Input: part model. Units: mm. Frame: model coordinates. A direction names the side the tool comes from. Round coordinates to 2 decimals unless told otherwise and drop trailing zeros. Loops run counter-clockwise (first coordinate to the right, second up) from the corner with the lowest first, then second, coordinate; pieces in that order, holes last. Notation, with made-up numbers: (-31.75, 56.25) -> (-1.75, 56.25) arc R31 cw to (-1.75, 89.25) -> close; hole circle Ø8 at (9.25, 55). An arc over 180 degrees is marked (long way). One line per question, with ' | ' between items. Start each with the question number.
Q1. Cut plane C-C on x = -23. Return loops of the section in (y, z), and give its area (3 significant figures).
Q2. Access query for faces 5 (the face through (114, 12.7, 1)), 6 (the face through (-1, 20, 38.1)), 7 (the face through (2, 0, 1)), 8 (the face through (-114, 12.7, 1)). Directions: +Z, -Z, +X, -X, +Y, -Y. A direction counts if a zero-diameter tool reaches every point of the face in a straight line with its end or side. Return the directions, or none.
Q3. Material intervals for L1, parallel to X at y = 18, z = 0 (3 decimals); L2, parallel to Z at x = 95.25, y = 15.5 (3 decimals); L3, parallel to X at y = 19, z = -41, sorted ascending.
Q4. Cut plane B-B on z = 0. Return loops of the section in (x, y) (3 decimals), and give its area (3 significant figures).
Q5. Contact query for flat-ended pins moving along their axis: P1, Ø6.5, axis at y = 17, z = -33, coming from the +X side; P2, Ø7, axis at x = 96.5, z = -1, coming from the +Y side; P3, Ø1.9, axis at x = -94.5, z = 1, coming from the +Y side; P4, Ø8.5, axis at x = -76.2, z = 38.1, coming from the +Y side. Output: stop coordinate, or through.
Q6. Mould query, pull axis X, two halves, no side actions, for faces 1 (the face through (-2, 13, 101.6)), 2 (the face through (101.6, 19, -1)), 3 (the face through (-79.45, 19.77, -41.58)), 4 (the face through (-101.6, 19, -1)). Classes: pulls with the +X half, pulls with the -X half, needs draft (parallel to the pull), parting line crosses it, or undercut.
Q7. Cut plane A-A on x = 95.25. Return loops of the section in (y, z) (3 decimals).
Autodesk Inventor part; units mm, degrees
ref_plane "YZ Plane" through (0, 0, 0) normal (1, 0, 0) x (0, 1, 0)
ref_plane "XZ Plane" through (0, 0, 0) normal (0, 1, 0) x (-1, 0, 0)
ref_plane "XY Plane" through (0, 0, 0) normal (0, 0, 1) x (1, 0, 0)
sketch "Sketch1" plane through (0, 0, 0) normal (0, 1, 0) x (-1, 0, 0)
  line L0 (127, 101.6) -> (101.6, 101.6)
  line L1 (-127, 101.6) -> (-127, -101.6)
  line L2 (-127, -101.6) -> (-101.6, -101.6)
  line L3 (127, -101.6) -> (127, 101.6)
  line L4 (127, 101.6) -> (-127, -101.6) construction
  line L5 (-127, 101.6) -> (127, -101.6) construction
  line L6 (127, -101.6) -> (101.6, -101.6)
  line L7 (101.6, -101.6) -> (101.6, 101.6)
  line L8 (101.6, 101.6) -> (127, 101.6)
  line L9 (127, 101.6) -> (127, -101.6)
  line L10 (-127, -101.6) -> (-101.6, -101.6)
  line L11 (-101.6, -101.6) -> (-101.6, 101.6)
  line L12 (-101.6, 101.6) -> (-127, 101.6)
  line L13 (-127, 101.6) -> (-127, -101.6)
  line L14 (101.6, -101.6) -> (127, -101.6)
  line L15 (101.6, 101.6) -> (-101.6, 101.6)
  line L16 (-101.6, 101.6) -> (-127, 101.6)
  line L17 (-101.6, -101.6) -> (101.6, -101.6)
  point P0 (0, 0)
  dimension "d0" = 254
  dimension "d1" = 203.2
  dimension "d2" = 25.4
  dimension "d3" = 25.4
extrude "Extrusion1" add sketch "Sketch1" along normal blind 25.4 contours L7 L17 L11 L15
extrude "Extrusion2" add sketch "Sketch1" along normal blind 12.7 contours L3 L6 L7 L0 | L11 L2 L1 L12
sketch "Sketch2" plane through (0, 25.4, 0) normal (0, 1, 0) x (1, 0, 0)
  line L0 (-76.2, -38.1) -> (76.2, -38.1)
  line L1 (76.2, -38.1) -> (76.2, 38.1)
  line L2 (76.2, 38.1) -> (-76.2, 38.1)
  line L3 (-76.2, 38.1) -> (-76.2, -38.1)
  line L4 (-76.2, -38.1) -> (76.2, 38.1) construction
  line L5 (76.2, -38.1) -> (-76.2, 38.1) construction
  circle A0 centre (-76.2, 38.1) radius 4.7625
  circle A1 centre (76.2, 38.1) radius 4.7625
  circle A2 centre (76.2, -38.1) radius 4.7625
  circle A3 centre (-76.2, -38.1) radius 4.7625
  point P0 (0, 0)
  dimension "d8" = 152.4
  dimension "d9" = 76.2
  dimension "d10" = 9.525
  dimension "d11" = 9.525
  dimension "d12" = 9.525
  dimension "d13" = 9.525
extrude "Extrusion3" cut sketch "Sketch2" against normal blind 11.43
sketch "Sketch3" plane through (0, 25.4, 0) normal (0, 1, 0) x (1, 0, 0)
  circle A0 centre (-95.25, 0) radius 3.175
  line L0 (-76.2, -33.3375) -> (-76.2, 33.3375)
  point P0 (0, 0)
  dimension "d16" = 6.35
  dimension "d17" = 19.05
extrude "Extrusion4" cut sketch "Sketch3" against normal blind 12.7
mirror "Mirror1" about plane through (0, 0, 0) normal (1, 0, 0) of "Extrusion4"
equation "\"d11\" = d10"
equation "\"d12\" = d10"
equation "\"d13\" = d10"
properties part number "Case Jig"
Results:
1) outline: (0, -101.6) -> (25.4, -101.6) -> (25.4, -38.1) -> (13.97, -38.1) -> (13.97, 38.1) -> (25.4, 38.1) -> (25.4, 101.6) -> (0, 101.6) -> close | area: 4,290 mm^2
2) face 5: +Z, -Z, +X, +Y | face 6: +Y | face 7: +Z, -Z, +X, -X, -Y | face 8: +Z, -Z, -X, +Y
3) L1: -101.6 to -98.425, -92.075 to -76.2, 76.2 to 92.075, 98.425 to 101.6 | L2: -101.6 to -3.175, 3.175 to 101.6 | L3: -101.6 to -79.98, -72.42 to 72.42, 79.98 to 101.6
4) outline: (-127, 0) -> (127, 0) -> (127, 12.7) -> (101.6, 12.7) -> (101.6, 25.4) -> (98.425, 25.4) -> (98.425, 12.7) -> (92.075, 12.7) -> (92.075, 25.4) -> (76.2, 25.4) -> (76.2, 13.97) -> (-76.2, 13.97) -> (-76.2, 25.4) -> (-92.075, 25.4) -> (-92.075, 12.7) -> (-98.425, 12.7) -> (-98.425, 25.4) -> (-101.6, 25.4) -> (-101.6, 12.7) -> (-127, 12.7) -> close | area: 3,900 mm^2
5) P1: x = 101.6 | P2: y = 25.4 | P3: y = 12.7 | P4: y = 13.97
6) face 1: needs draft | face 2: pulls with the +X half | face 3: undercut | face 4: pulls with the -X half
7) outline: (0, -101.6) -> (25.4, -101.6) -> (25.4, -3.175) -> (12.7, -3.175) -> (12.7, 3.175) -> (25.4, 3.175) -> (25.4, 101.6) -> (0, 101.6) -> close
